Design review of the part built by this model. Coordinates are the model's own, in mm. Face numbers are marked on the shaded views. A direction names the side the tool comes from. Give positions to 0.01 mm unless a question says otherwise; leave off trailing zeros. Write each loop counter-clockwise with the first axis right and the second up, starting at its lowest first coordinate (ties: lowest second). Pieces come first, ordered by that corner, then holes. Notation, with made-up numbers: M 54,9 L 113,9 A30 ccw 113,38 Z; hole C -7,32.25 d11. An arc over 180 degrees is marked long. One line per item, written item: value. Start each with the question number.
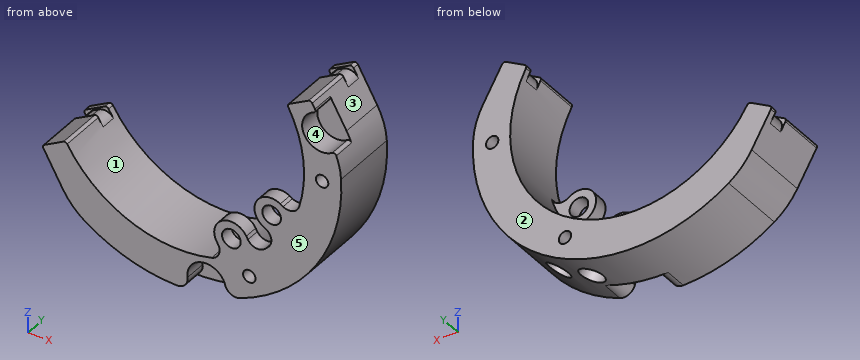
```python
from build123d import *

# Parameters (mm, degrees)
BOSS_EXTRUDE1_DEPTH                        = 15.367
BOSS_EXTRUDE2_DEPTH                        = 3.175
F_8_CLEARANCE_HOLE1_D                      = 4.3053
SKETCH10_R                                 = 4.445
CUT_EXTRUDE2_DEPTH                         = 5.08
FILLET3_R                                  = 2.54
SKETCH12_W                                 = 0.381
SKETCH12_H                                 = 3.429
CUT_EXTRUDE5_DEPTH                         = 80.383868095
FILLET6_R                                  = 2.54
CBORE_START                                = -39
CBORE_FOR_4_SOCKET_HEAD_CAP_SCREW1_OUTL_R  = 2.77876
CBORE_FOR_4_SOCKET_HEAD_CAP_SCREW1_DEPTH   = 4.004980035
CBORE_START_2                              = -34.995019965
CBORE_FOR_4_SOCKET_HEAD_CAP_SCREW1_2_OU_R  = 1.4732
CBORE_FOR_4_SOCKET_HEAD_CAP_SCREW1_2_DEPTH = 6.995019965
CUT_EXTRUDE6_REACH                         = 58.03
SKETCH17_R                                 = 1.4351
FILLET7_R                                  = 0.635
CUT_EXTRUDE7_DEPTH                         = 61.777907815


with BuildPart() as part:
    # Sketch1 → Boss-Extrude1 (new body)
    with BuildSketch(Plane(origin=(0, 0, 0), x_dir=(1, 0, 0), z_dir=(0, 1, 0))):
        with BuildLine():
            Line((-35.805540197, 9.673815643), (-31.043040197, 17.922707614))
            Line((-31.043040197, 17.922707614), (-25.543778883, 14.747707614))
            ThreePointArc((-25.543778883, 14.747707614), (-14.747707614, -25.543778883), (25.543778883, -14.747707614))
            Line((25.543778883, -14.747707614), (31.043040197, -17.922707614))
            Line((31.043040197, -17.922707614), (26.280540197, -26.171599585))
            ThreePointArc((26.280540197, -26.171599585), (23.947229931, -29.306716595), (20.954526486, -31.820085162))
            ThreePointArc((20.954526486, -31.820085162), (-19.05, -32.995567884), (-38.034265344, 2.23710968))
            ThreePointArc((-38.034265344, 2.23710968), (-37.353976038, 6.085551173), (-35.805540197, 9.673815643))
        make_face()
    extrude(amount=BOSS_EXTRUDE1_DEPTH)

    # Sketch8 → Boss-Extrude2 (add)
    with BuildSketch(Plane(origin=(0, 0, 0), x_dir=(1, 0, 0), z_dir=(0, 1, 0))):
        with BuildLine():
            Line((-9.262961679, -23.981420256), (-11.176555889, -27.295862653))
            ThreePointArc((-11.176555889, -27.295862653), (-14.747707614, -25.543778883), (-18.050632531, -23.327112653))
            Line((-18.050632531, -23.327112653), (-16.137038321, -20.012670256))
            ThreePointArc((-16.137038321, -20.012670256), (-10.715625, -18.560006935), (-9.262961679, -23.981420256))
        make_face()
        with BuildLine():
            Line((3.96875, -25.4), (3.96875, -29.22718842))
            ThreePointArc((3.96875, -29.22718842), (0, -29.495415229), (-3.96875, -29.22718842))
            Line((-3.96875, -29.22718842), (-3.96875, -25.4))
            ThreePointArc((-3.96875, -25.4), (0, -21.43125), (3.96875, -25.4))
        make_face()
    extrude(amount=BOSS_EXTRUDE2_DEPTH)

    # #8 Clearance Hole1 (through all)
    with Locations(Plane(origin=(0, 3.175, 0), x_dir=(1, 0, 0), z_dir=(0, 1, 0))):
        with Locations((0, -25.4), (-12.7, -21.997045256)):
            Hole(F_8_CLEARANCE_HOLE1_D / 2)

    # Sketch10 → Cut-Extrude2 (cut)
    with BuildSketch(Plane.XZ):
        with Locations((-26.502210802, 23.360731753)):
            Circle(SKETCH10_R)
        with Locations((26.502210802, 23.360731753)):
            Circle(SKETCH10_R)
    extrude(amount=-CUT_EXTRUDE2_DEPTH, mode=Mode.SUBTRACT)

    # Fillet3
    fillet3_edges = [part.edges().sort_by_distance(p)[0] for p in [
        (-18.050632531, 1.5875, 23.327112653),
        (-11.176555889, 1.5875, 27.295862653),
        (-3.96875, 1.5875, 29.22718842),
        (3.96875, 1.5875, 29.22718842),
        (-30.836833913, 2.54, 22.376319497),
        (-26.069605371, 2.54, 27.784630208),
    ]]
    fillet(fillet3_edges, radius=FILLET3_R)

    # Sketch12 → Cut-Extrude5 (cut, through all)
    with BuildSketch(Plane(origin=(31.043040197, 0, 17.922707614), x_dir=(0.5000000000000004, 0, -0.8660254037844384), z_dir=(0.8660254037844384, 0, 0.5000000000000004))):
        with Locations((-0.1905, 12.192)):
            Rectangle(SKETCH12_W, SKETCH12_H)
    extrude(amount=-CUT_EXTRUDE5_DEPTH, mode=Mode.SUBTRACT)

    # Fillet6
    fillet6_edges = [part.edges().sort_by_distance(p)[0] for p in [
        (-25.732147733, 12.192, -14.416521515),
        (25.351147733, 12.192, 15.076432873),
        (-31.233540197, 12.192, -17.592751936),
        (30.852540197, 12.192, 18.252663293),
    ]]
    fillet(fillet6_edges, radius=FILLET6_R)

    # CBORE for #4 Socket Head Cap Screw1: read off the stored shape, not the designer's step
    # CBORE for #4 Socket Head Cap Screw1 outl → CBORE for #4 Socket Head Cap Screw1 (cut)
    with BuildSketch(Plane(origin=(0, 0, 0), x_dir=(0.8660254037844374, 0, 0.5000000000000022), z_dir=(0.5000000000000022, 0, -0.8660254037844374)).offset(CBORE_START)):
        with Locations((4.445, -8.89)):
            Circle(CBORE_FOR_4_SOCKET_HEAD_CAP_SCREW1_OUTL_R)
        with Locations((-4.445, -8.89)):
            Circle(CBORE_FOR_4_SOCKET_HEAD_CAP_SCREW1_OUTL_R)
    extrude(amount=CBORE_FOR_4_SOCKET_HEAD_CAP_SCREW1_DEPTH, mode=Mode.SUBTRACT)

    # CBORE for _4 Socket Head Cap Screw1 2 ou → CBORE for _4 Socket Head Cap Screw1 2 (cut)
    with BuildSketch(Plane(origin=(0, 0, 0), x_dir=(0.8660254037844374, 0, 0.5000000000000022), z_dir=(0.5000000000000022, 0, -0.8660254037844374)).offset(CBORE_START_2)):
        with Locations((4.445, -8.89)):
            Circle(CBORE_FOR_4_SOCKET_HEAD_CAP_SCREW1_2_OU_R)
        with Locations((-4.445, -8.89)):
            Circle(CBORE_FOR_4_SOCKET_HEAD_CAP_SCREW1_2_OU_R)
    extrude(amount=CBORE_FOR_4_SOCKET_HEAD_CAP_SCREW1_2_DEPTH, mode=Mode.SUBTRACT)

    # Sketch17 → Cut-Extrude6 (cut, up to next)
    with BuildSketch(Plane(origin=(0, 15.367, 0), x_dir=(1, 0, 0), z_dir=(0, 1, 0)), mode=Mode.PRIVATE) as cut_extrude6_sk1:
        with Locations(Location((-16.8275, -29.146084964, 0), (0, 0, 270))):
            Circle(SKETCH17_R)
    cut_extrude6_tool1 = extrude(cut_extrude6_sk1.sketch, amount=-CUT_EXTRUDE6_REACH, mode=Mode.PRIVATE) & part.part
    # Sketch17 → Cut-Extrude6 (cut, up to next)
    with BuildSketch(Plane(origin=(0, 15.367, 0), x_dir=(1, 0, 0), z_dir=(0, 1, 0)), mode=Mode.PRIVATE) as cut_extrude6_sk2:
        with Locations(Location((16.8275, -29.146084964, 0), (0, 0, 270))):
            Circle(SKETCH17_R)
    cut_extrude6_tool2 = extrude(cut_extrude6_sk2.sketch, amount=-CUT_EXTRUDE6_REACH, mode=Mode.PRIVATE) & part.part
    add(cut_extrude6_tool1.solids().sort_by_distance((-16.8275, 15.367, 29.146085))[0], mode=Mode.SUBTRACT)
    add(cut_extrude6_tool2.solids().sort_by_distance((16.8275, 15.367, 29.146085))[0], mode=Mode.SUBTRACT)

    # Fillet7
    fillet7_edges = [part.edges().sort_by_distance(p)[0] for p in [
        (25.543778883, 5.23875, 14.747707614),
        (31.043040197, 5.23875, 17.922707614),
        (25.543778883, 14.63675, 14.747707614),
        (31.043040197, 14.63675, 17.922707614),
        (-31.043040197, 5.23875, -17.922707614),
        (-25.543778883, 5.23875, -14.747707614),
        (-31.043040197, 14.63675, -17.922707614),
        (-25.543778883, 14.63675, -14.747707614),
        (25.323084778, 2.54, 27.646485691),
        (29.691178841, 2.54, 20.264200169),
    ]]
    fillet(fillet7_edges, radius=FILLET7_R)


with BuildPart() as body_2:
    # Mirror4: mirrored copy
    add(part.part.mirror(Plane(origin=(1.27, 0, -2.199704526), x_dir=(0.8660254037844389, 0, 0.49999999999999944), z_dir=(0.49999999999999967, 0, -0.8660254037844389))))


with BuildPart() as part_1:
    add(part.part)

    # Sketch18 → Cut-Extrude7 (cut, through all)
    with BuildSketch(Plane(origin=(0, 15.367, 0), x_dir=(1, 0, 0), z_dir=(0, 1, 0))):
        Polygon((-35.598010153, 20.561277362), (38.427739113, -19.56618359), (10.396462238, -40.426668706), (-26.181818955, -37.529379107), (-44.652040151, -8.121889672), align=None)
    extrude(amount=-CUT_EXTRUDE7_DEPTH, mode=Mode.SUBTRACT)


solid = body_2.part
```
Q1. Wall thickness on line 1 (X direction, y = 1.5, z = -27.5); line 2 (Y direction, x = 12.5, z = -38.5); line 3 (Z direction, x = 35.5, y = 1.5) (3 decimals): over which ranges is each line inside the solid? List them lowest first. Write a range as from..to.
Q2. Take a section at D-D, the plane z = -9. Give the boundary of the cut face in (x, y).
Q3. The part is to be moulded in two halves that separate along X. For the marked faces 1, 2 and 3, say which applies: pulls with the +X half, pulls with the -X half, needs draft (parallel to the pull), parting line crosses it, or undercut.
Q4. Take a section at A-A, the plane y = 13. Give the boundary of the cut face in (x, z) (1 decimal).
Q5. Take a section at C-C, the plane x = 0.5. Give the boundary of the cut face in (y, z).
Q6. Machinability: for the marked faces 4 and 5, which of the approach directions +Z, -Z, +X, -X, +Y, -Y give a long, thin tool a straight path to every point of the face, cutting with its end or side? Answer none if there is none.
Q7. Take a section at B-B, the plane y = 2.25. State how many separate pieces and enclosed holes the cut face has, then the cut area to 3 significant figures.
Q8. For P1, Ø7, axis at x = 36.02, z = 6.87, coming from the -Y side; P2, Ø2, axis at y = 12.5, z = 3.5, coming from the -X side; P3, Ø5.5, axis at x = 15.24, z = -26.4, coming from the +Y side (3 decimals), all flat-tipped, find the tip position at first contact; note any pin that passes through.
Results list:
1. line 1: x = -25.51..-15.8, 11.43..13.39, 17.09..32.84
1. line 2: y = 5.08..15.37
1. line 3: z = -23.511..-5.655, -3.144..2.458
2. outline: M 31.67,0 L 40.36,0 L 40.36,15.37 L 31.67,15.37 Z
3. face 1: undercut
3. face 2: needs draft
3. face 3: pulls with the +X half
4. outline: M -27,-24.9 L -23.7,-30.6 A16.9 ccw -18.4,-36.2 A38.1 ccw 40.6,-2.2 A16.9 ccw 38.3,5.3 L 35,11 A2.5 ccw 31.6,11.9 L 30.4,11.2 A2.5 ccw 29.3,8 A29.5 cw -21.6,-21.4 A2.5 ccw -24.9,-20.7 L -26.1,-21.4 A2.5 ccw Z; hole C 19.4,-33.5 d2.9; hole C 36.2,-4.4 d2.9
5. outline: M 0,-42.44 L 15.37,-42.44 L 15.37,-33.82 L 0,-33.82 Z
6. face 4: -Y
6. face 5: +Z, -Z, +X, -X, -Y
7. separate pieces: 1
7. enclosed holes: 4
7. area: 852 mm^2
8. P1: stops at y = 5.08
8. P2: stops at x = 30.66
8. P3: stops at y = 3.175
